Geometry check sheet. Reference: drawing and pictorial views, mm from the part's lowest x, y, z. A direction names the side the tool comes from. Give positions to 0.01 mm unless a question says otherwise; leave off trailing zeros. Loops run counter-clockwise (first coordinate to the right, second up) from the corner with the lowest first, then second, coordinate; pieces in that order, holes last. Notation, with made-up numbers: (36.5, 63.25) - (73.5, 63.25) arc R23 ccw to (73.5, 99.25) - close; hole circle Ø10 at (-21.75, 50). An arc over 180 degrees is marked (long way). Answer in a Markdown table with one row per item. Add a question column.
(1) Go/stop test with flat-tipped pins: P1, Ø4.5, axis at x = 10, y = 18.05, coming from the -Z side; P2, Ø0.9, axis at y = 32.5, z = 1, coming from the -X side; P3, Ø11, axis at x = 64.5, y = 17, coming from the +Z side; P4, Ø16, axis at y = 15.5, z = 37, coming from the -X side. Record where each tip stops, or that it passes through.
(2) Set-up check for the marked faces 1, 2 and 3: record each of +Z, -Z, +X, -X, +Y, -Y from which the full face is reachable in a straight line by a thin tool's end or side.
(3) Thickness scan on L1, parallel to Y at x = 10, z = 54.45; L2, parallel to Z at x = 60, y = 25.5; L3, parallel to Z at x = 12, y = 12.5. Record the ranges inside material, lowest first.
(4) Sectioned sample at D-D on y = 6.5. Enter the section's corners in (x, z).
(5) Sectioned sample at B-B on x = 25. Enter the section's corners in (y, z).
(6) Sectioned sample at C-C on z = 29.5. Enter the section's corners in (x, y).
(7) Sectioned sample at A-A on y = 18.05. Enter the section's corners in (x, z).
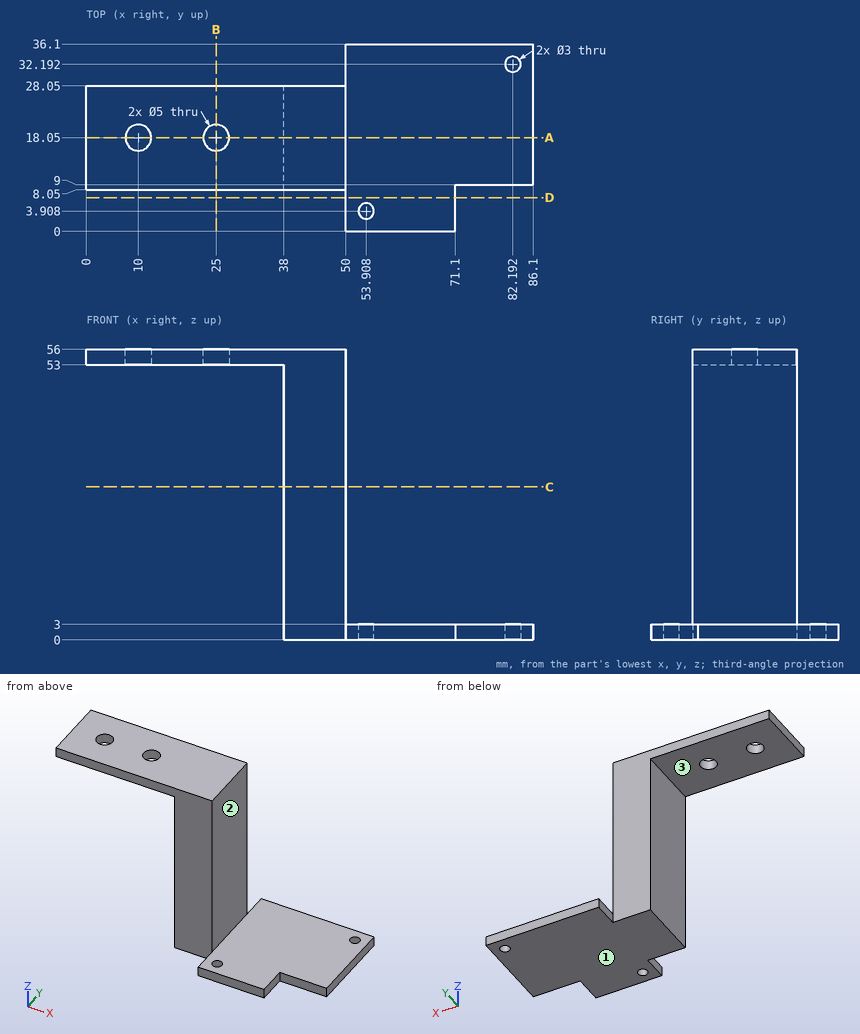
Reply:
| question | item | result |
|---|---|---|
| 1 | P1 | through |
| 1 | P2 | x = 50 |
| 1 | P3 | z = 3 |
| 1 | P4 | x = 38 |
| 2 | face 1 | -Z, +X, -X, +Y, -Y |
| 2 | face 2 | +Z, +X, +Y, -Y |
| 2 | face 3 | -Z, -X, +Y, -Y |
| 3 | L1 | 8.05 to 15.55, 20.55 to 28.05 |
| 3 | L2 | 0 to 3 |
| 3 | L3 | 53 to 56 |
| 4 | outline | (50, 0) - (71.1, 0) - (71.1, 3) - (50, 3) - close |
| 5 | outline | (8.05, 53) - (15.55, 53) - (15.55, 56) - (8.05, 56) - close; (20.55, 53) - (28.05, 53) - (28.05, 56) - (20.55, 56) - close |
| 6 | outline | (38, 8.05) - (50, 8.05) - (50, 28.05) - (38, 28.05) - close |
| 7 | outline | (0, 53) - (7.5, 53) - (7.5, 56) - (0, 56) - close; (12.5, 53) - (22.5, 53) - (22.5, 56) - (12.5, 56) - close; (27.5, 53) - (38, 53) - (38, 0) - (86.1, 0) - (86.1, 3) - (50, 3) - (50, 56) - (27.5, 56) - close |
